Geometry: final body of the model. Coordinates: model frame, mm. A direction names the side the tool comes from. Round coordinates to 2 decimals unless told otherwise and drop trailing zeros. Loops run counter-clockwise (first coordinate to the right, second up) from the corner with the lowest first, then second, coordinate; pieces in that order, holes last. Notation, with made-up numbers: (6.5, 8) - (47.5, 8) arc R9 ccw to (47.5, 15) - close; hole circle Ø3 at (33, -0.75). An arc over 180 degrees is marked (long way). Answer as CSV lines item,"result".
from build123d import *

# Parameters (mm, degrees)
F1_DEPTH = 20
F3_D     = 10


with BuildPart() as f1:
    # F0 (on Front) → F1 (new body, symmetric)
    with BuildSketch(Plane.XZ):
        Polygon((0, 60), (0, 0), (40, 0), (40, 5), (5, 5), (5, 60), align=None)
    extrude(amount=F1_DEPTH, both=True)

    # F3 (through all)
    with Locations(Plane.XY.offset(5)):
        with Locations((25, 0)):
            Hole(F3_D / 2)


solid = f1.part
(1) Draft query along Y for faces 3 (the face through (30, 0, 2)), 4 (the face through (0, 0, 30)), 5 (the face through (4, 20, 21)). Return one class per face: pulls with the +Y half, pulls with the -Y half, needs draft (parallel to the pull), parting line crosses it, or undercut.
Findings below:
face 3,"undercut"
face 4,"needs draft"
face 5,"pulls with the +Y half"
(2) Material intervals for line 1 along Y through (x, z) = (25, 3); line 2 along X through (y, z) = (-13, 7.5), sorted ascending.
Findings below:
line 1,"-20 to -5, 5 to 20"
line 2,"0 to 5"
(3) Section D-D (z = 31). Output: boundary loops of the cut face in (x, y).
Findings below:
outline,"(0, -20) - (5, -20) - (5, 20) - (0, 20) - close"
(4) Section A-A (x = 25). Output: boundary loops of the cut face in (y, z).
Findings below:
outline,"(-20, 0) - (-5, 0) - (-5, 5) - (-20, 5) - close; (5, 0) - (20, 0) - (20, 5) - (5, 5) - close"
(5) Access query for faces 1 (the face through (19, 0, 5)), 2 (the face through (40, 0, 2)). Directions: +Z, -Z, +X, -X, +Y, -Y. A direction counts if a zero-diameter tool reaches every point of the face in a straight line with its end or side. Return the directions, or none.
Findings below:
face 1,"+Z, +X, +Y, -Y"
face 2,"+Z, -Z, +X, +Y, -Y"
(6) Section C-C (y = -9). Output: boundary loops of the cut face in (x, z).
Findings below:
outline,"(0, 0) - (40, 0) - (40, 5) - (5, 5) - (5, 60) - (0, 60) - close"
(7) Section B-B (y = 4). Output: boundary loops of the cut face in (x, z), and give its area (3 significant figures).
Findings below:
outline,"(0, 0) - (22, 0) - (22, 5) - (5, 5) - (5, 60) - (0, 60) - close; (28, 0) - (40, 0) - (40, 5) - (28, 5) - close"
area,"445 mm2"
(8) Pin query (flat end, axial travel): P1, Ø8, axis at x = 19, y = 1, coming from the +Z side. Return the tip coordinate at first contact, or that it passes through.
Findings below:
P1,"z = 5"
